The model under review builds one solid part; all positions refer to its coordinate system, in mm. Round coordinates to 2 decimals unless told otherwise and drop trailing zeros. Order: outer loops, then holes, each group sorted by start corner. A loop starts at its lowest first (then second) coordinate and runs counter-clockwise, first axis right, second up.
from build123d import *

# Parameters (mm, degrees)
SKETCH1_R               = 1.5875
BOSS_EXTRUDE1_DEPTH     = 95.25
F_1_4_20_TAPPED_HOLE2_D = 5.1054


with BuildPart() as part:
    # Sketch1 → Boss-Extrude1 (new body)
    with BuildSketch(Plane.XY):
        with BuildLine():
            Line((-4.430514159, -4.283916762), (-3.451917569, -5.978896013))
            Line((-3.451917569, -5.978896013), (-1.49472801, -5.978896013))
            ThreePointArc((-1.49472801, -5.978896013), (-3.62e-07, -4.484168365), (1.49472801, -5.978896013))
            Line((1.49472801, -5.978896013), (3.451916913, -5.978896013))
            Line((3.451916913, -5.978896013), (4.430513537, -4.28391694))
            ThreePointArc((4.430513537, -4.28391694), (3.883406572, -2.242085948), (5.925237563, -1.694978983))
            Line((5.925237563, -1.694978983), (6.903834188, 9.1e-08))
            Line((6.903834188, 9.1e-08), (5.925237797, 1.694979115))
            ThreePointArc((5.925237797, 1.694979115), (3.883406856, 2.242086266), (4.430514007, 4.283917207))
            Line((4.430514007, 4.283917207), (3.451917569, 5.978896313))
            Line((3.451917569, 5.978896313), (1.494720042, 5.978896313))
            ThreePointArc((1.494720042, 5.978896313), (3.62e-07, 4.484176634), (-1.494720042, 5.978896313))
            Line((-1.494720042, 5.978896313), (-3.451916913, 5.978896313))
            Line((-3.451916913, 5.978896313), (-4.43051364, 4.283917299))
            ThreePointArc((-4.43051364, 4.283917299), (-3.883406799, 2.242086274), (-5.925237823, 1.694979433))
            Line((-5.925237823, 1.694979433), (-6.90383455, 4.18e-07))
            Line((-6.90383455, 4.18e-07), (-5.925238028, -1.694978715))
            ThreePointArc((-5.925238028, -1.694978715), (-3.88340707, -2.242085804), (-4.430514159, -4.283916762))
        make_face()
        Circle(SKETCH1_R, mode=Mode.SUBTRACT)
    extrude(amount=-BOSS_EXTRUDE1_DEPTH)

    # 1/4-20 Tapped Hole2 (through all)
    with Locations(Plane.XY):
        with Locations((0, 0)):
            Hole(F_1_4_20_TAPPED_HOLE2_D / 2)


solid = part.part
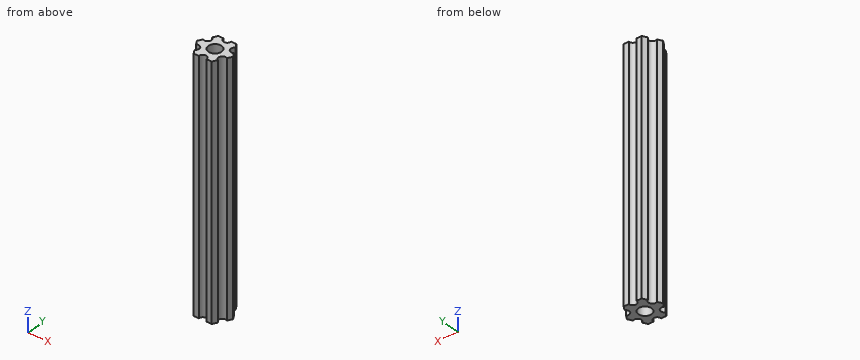
(1) We need section B-B (z = -69). Give the boundary of the cut face in (x, y), and give its area (3 significant figures).
(2) We need section A-A (x = 0). Give the boundary of the cut face in (y, z).
(3) To check wall thickness, follow L1, parallel to Y at x = 0, z = -71; L2, parallel to X at y = -2.75, z = -30; L3, parallel to Y at x = 2, z = -65.5. State the ranges of each line that lie inside material, in increasing order.
(4) We need section C-C (y = 3.5). Give the boundary of the cut face in (x, z), and give its area (3 significant figures).
(5) Clearance check with flat-ended pins moving along their axes: P1, Ø3, axis at x = 5, z = -15.5, coming from the +Y side; P2, Ø2, axis at y = 2.5, z = -64.5, coming from the -X side; P3, Ø4, axis at y = 2.5, z = -52.5, coming from the -X side. State where each tip first meets the part, or that it passes through.
Verdict:
1. outline: (-6.9, 0) - (-5.93, -1.69) arc R1.49 cw to (-4.43, -4.28) - (-3.45, -5.98) - (-1.49, -5.98) arc R1.49 cw to (1.49, -5.98) - (3.45, -5.98) - (4.43, -4.28) arc R1.49 cw to (5.93, -1.69) - (6.9, 0) - (5.93, 1.69) arc R1.49 cw to (4.43, 4.28) - (3.45, 5.98) - (1.49, 5.98) arc R1.49 cw to (-1.49, 5.98) - (-3.45, 5.98) - (-4.43, 4.28) arc R1.49 cw to (-5.93, 1.69) - close; hole circle Ø5.11 at (0, 0)
1. area: 82.3 mm2
2. outline: (-4.48, -95.25) - (-2.55, -95.25) - (-2.55, 0) - (-4.48, 0) - close; (2.55, -95.25) - (4.48, -95.25) - (4.48, 0) - (2.55, 0) - close
3. L1: y = -4.48 to -2.55, 2.55 to 4.48
3. L2: x = -3.7 to 3.7
3. L3: y = -5.98 to -1.59, 1.59 to 5.98
4. outline: (-3.77, -95.25) - (3.77, -95.25) - (3.77, 0) - (-3.77, 0) - close
4. area: 719 mm2
5. P1: stops at y = 5.9
5. P2: stops at x = -6.04
5. P3: stops at x = -6.62
